```python
from build123d import *

# Parameters (mm, degrees)
BOSS_EXTRUDE1_DEPTH                     = 40
CBORE_FOR_M5_HEX_HEAD_BOLT3_D           = 5.5
CBORE_FOR_M5_HEX_HEAD_BOLT3_CBORE_D     = 12.24
CBORE_FOR_M5_HEX_HEAD_BOLT3_CBORE_DEPTH = 3.58


with BuildPart() as part:
    # Sketch1 → Boss-Extrude1 (new body)
    with BuildSketch(Plane.XY):
        with BuildLine():
            Line((0, 0), (300, 0))
            ThreePointArc((300, 0), (320, 20), (300, 40))
            Line((300, 40), (0, 40))
            ThreePointArc((0, 40), (-23.145502494, 43.660770159), (-44.031528593, 54.285714286))
            ThreePointArc((-44.031528593, 54.285714286), (-34.948942351, 16.652664524), (0, 0))
        make_face()
    extrude(amount=BOSS_EXTRUDE1_DEPTH)

    # CBORE for M5 Hex Head Bolt3 (through all)
    with Locations(Plane(origin=(0, 0, 0), x_dir=(-1, 0, 0), z_dir=(0, -1, 0))):
        with Locations((-260, -15), (-260, -25), (-200, -25), (-200, -15)):
            CounterBoreHole(CBORE_FOR_M5_HEX_HEAD_BOLT3_D / 2, CBORE_FOR_M5_HEX_HEAD_BOLT3_CBORE_D / 2, CBORE_FOR_M5_HEX_HEAD_BOLT3_CBORE_DEPTH)


solid = part.part
```
Geometry: final body of the model. Coordinates: model frame, mm. A direction names the side the tool comes from. Coordinates: 2 decimals unless noted, no trailing zeros. Write each loop counter-clockwise with the first axis right and the second up, starting at its lowest first coordinate (ties: lowest second). Pieces come first, ordered by that corner, then holes. Notation, with made-up numbers: M 62.25,17.25 L 66.25,17.25 A15 ccw 66.25,32.25 Z; hole C 66,23.25 d9. An arc over 180 degrees is marked long. Answer as CSV lines item,"result". Start each with the question number.
Q1. Mould query, pull axis X, two halves, no side actions, for faces 4 (the cylindrical face through (200.216, 1.765, 31.116)), 5 (the flat face through (135, 21, 40)), 6 (the cylindrical face through (-22.83, 43.56, 19.72)). Classes: released by +X, released by -X, zero draft, split by the parting line, or undercut.
Q2. Cut plane C-C on x = -21.5. Return the cut outline in (y, z).
Q3. Line query: line 1 (Z direction, x = 260, y = 31); line 2 (X direction, y = 15, z = 15); line 3 (X direction, y = 11, z = 16.5). Output: solid intervals per line, ascending. Write a range as from..to.
Q4. Reachability of faces 1 (the flat face through (148, 0, 20)), 2 (the flat face through (152, 40, 20)), 3 (the cylindrical face through (259.784, 1.765, 8.884)) from +Z, -Z, +X, -X, +Y, -Y: full face, straight path, thin tool, end or side. Return the list, or none.
Q5. Cut plane B-B on x = 43.5. Return the cut outline in (y, z), then the cut area to 3 significant figures.
Q6. Cut plane A-A on y = 12. Return the cut outline in (x, z), then the cut area to 3 significant figures.
Q7. Pin query (flat end, axial travel): P1, Ø10, axis at x = 260, z = 25, coming from the -Y side; P2, Ø1, axis at y = 33, z = 26, coming from the -X side; P3, Ø12, axis at x = 204, z = 13.5, coming from the +Y side; P4, Ø3, axis at x = 237, z = 15.5, coming from the -Y side. Return the tip coordinate at first contact, or that it passes through.
Findings below:
1,face 4,"undercut"
1,face 5,"zero draft"
1,face 6,"released by +X"
2,outline,"M 5.47,0 L 43.15,0 L 43.15,40 L 5.47,40 Z"
3,line 1,"z = 0..12.25, 17.75..22.25, 27.75..40"
3,line 2,"x = -33.54..197.25, 202.75..257.25, 262.75..319.36"
3,line 3,"x = -29.48..197.7, 202.3..257.7, 262.3..317.86"
4,face 1,"+Z, -Z, +X, -X, -Y"
4,face 2,"+Z, -Z, +X, +Y"
4,face 3,"-Y"
5,outline,"M 0,0 L 40,0 L 40,40 L 0,40 Z"
5,area,"1,600 mm2"
6,outline,"M -30.59,0 L 318.33,0 L 318.33,40 L -30.59,40 Z; hole C 200,15 d5.5; hole C 200,25 d5.5; hole C 260,15 d5.5; hole C 260,25 d5.5"
6,area,"13,900 mm2"
7,P1,"stops at y = 3.58"
7,P2,"stops at x = -43.51"
7,P3,"stops at y = 40"
7,P4,"stops at y = 0"
